Part model, mm, in its own coordinate system. Coordinates: 2 decimals unless noted, no trailing zeros. Order: outer loops, then holes, each group sorted by start corner. A loop starts at its lowest first (then second) coordinate and runs counter-clockwise, first axis right, second up. Notation, with made-up numbers: (-4, 64) - (51, 64) arc R15 cw to (51, 69) - close; hole circle Ø5 at (3.25, 24). An arc over 180 degrees is marked (long way). Use a Markdown table: item, result. Add a question column.
1) Saw through at D-D on y = 2.55. Count the separate pieces of the cut face and the enclosed holes in it, then the cut area to 3 significant figures.
2) Saw through at C-C on x = -42. List the corners of the cut face in (y, z).
3) Saw through at B-B on z = 20. List the corners of the cut face in (x, y), then the cut area to 3 significant figures.
4) Wall check: L1, parallel to Z at x = 22, y = 0.15; L2, parallel to X at y = 0.8, z = 25.5; L3, parallel to X at y = 2.4, z = -24. Give the ranges that are in metal, low to high. Write a range as [from, to].
5) Saw through at A-A on x = 22. List the corners of the cut face in (y, z).
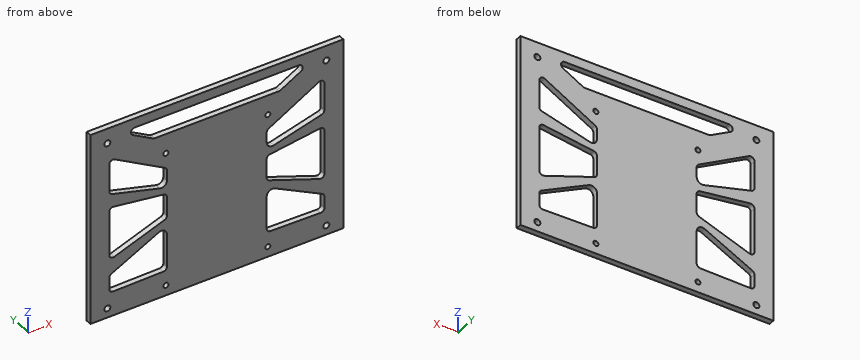
```python
from build123d import *

# Parameters (mm, degrees)
SKETCH_1_W          = 134
SKETCH_1_H          = 103
EXTRUDE_1_DEPTH     = 3
SKETCH_5_R          = 1.35
CUT_EXTRUDE_3_DEPTH = 85.559150895
SKETCH_6_R          = 1.6
CUT_EXTRUDE_4_DEPTH = 85.559150895
CUT_EXTRUDE_5_DEPTH = 85.559150895
FILLET_1_R          = 3
CUT_EXTRUDE_6_DEPTH = 85.559150895
FILLET_2_R          = 2


with BuildPart() as part:
    # 草图1 → 凸台-拉伸1 (new body)
    with BuildSketch(Plane(origin=(0, 0, 0), x_dir=(1, 0, 0), z_dir=(0, 1, 0))):
        Rectangle(SKETCH_1_W, SKETCH_1_H)
    extrude(amount=EXTRUDE_1_DEPTH)

    # 草图5 → 切除-拉伸3 (cut, through all)
    with BuildSketch(Plane(origin=(0, 3, 0), x_dir=(1, 0, 0), z_dir=(0, 1, 0))):
        with Locations(Location((27, -26, 0), (0, 0, 270))):
            Circle(SKETCH_5_R)
        with Locations(Location((-27, -26, 0), (0, 0, 270))):
            Circle(SKETCH_5_R)
        with Locations(Location((27, 46, 0), (0, 0, 270))):
            Circle(SKETCH_5_R)
        with Locations(Location((-27, 46, 0), (0, 0, 270))):
            Circle(SKETCH_5_R)
    extrude(amount=-CUT_EXTRUDE_3_DEPTH, mode=Mode.SUBTRACT)

    # 草图6 → 切除-拉伸4 (cut, through all)
    with BuildSketch(Plane(origin=(0, 3, 0), x_dir=(1, 0, 0), z_dir=(0, 1, 0))):
        with Locations(Location((58, 46.5, 0), (0, 0, 270))):
            Circle(SKETCH_6_R)
        with Locations(Location((58, -43.5, 0), (0, 0, 270))):
            Circle(SKETCH_6_R)
        with Locations(Location((-58, 46.5, 0), (0, 0, 90))):
            Circle(SKETCH_6_R)
        with Locations(Location((-58, -43.5, 0), (0, 0, 90))):
            Circle(SKETCH_6_R)
    extrude(amount=-CUT_EXTRUDE_4_DEPTH, mode=Mode.SUBTRACT)

    # 草图7 → 切除-拉伸5 (cut, through all)
    with BuildSketch(Plane.XZ):
        Polygon((-26.4206829, 17.634605341), (-57, 34.897123059), (-57, 15.273103969), (-26.4206829, 7.079400646), align=None)
        Polygon((-26.4206829, 3.713184828), (-57, 8.010827578), (-57, -20.746303353), (-26.4206829, -9.616342144), align=None)
        Polygon((-26.4206829, -37.989615661), (-26.4206829, -13.46201033), (-57, -29.042950621), (-57, -38.482830453), align=None)
        Polygon((57, -29.042950621), (26.4206829, -13.46201033), (26.4206829, -37.989615661), (57, -38.482830453), align=None)
        Polygon((26.4206829, 3.713184828), (26.4206829, -9.616342144), (57, -20.746303353), (57, 8.010827578), align=None)
        Polygon((26.4206829, 17.634605341), (26.4206829, 7.079400646), (57, 15.273103969), (57, 34.897123059), align=None)
    extrude(amount=-CUT_EXTRUDE_5_DEPTH, mode=Mode.SUBTRACT)

    # 圆角1
    fillet_1_edges = [part.edges().sort_by_distance(p)[0] for p in [
        (-26.4206829, 1.5, 7.079400646),
        (-26.4206829, 1.5, -13.46201033),
        (26.4206829, 1.5, -13.46201033),
        (26.4206829, 1.5, 7.079400646),
    ]]
    fillet(fillet_1_edges, radius=FILLET_1_R)

    # 草图9 → 切除-拉伸6 (cut, through all)
    with BuildSketch(Plane.XZ):
        Polygon((51.109101135, 46.5), (33.394815421, 36.5), (-33.394815421, 36.5), (-51.109101135, 46.5), align=None)
    extrude(amount=-CUT_EXTRUDE_6_DEPTH, mode=Mode.SUBTRACT)

    # 圆角2
    fillet_2_edges = [part.edges().sort_by_distance(p)[0] for p in [
        (-57, 1.5, 15.273103969),
        (-57, 1.5, 34.897123059),
        (-26.4206829, 1.5, 17.634605341),
        (-51.109101135, 1.5, 46.5),
        (51.109101135, 1.5, 46.5),
        (33.394815421, 1.5, 36.5),
        (-33.394815421, 1.5, 36.5),
        (-26.4206829, 1.5, -37.989615661),
        (-57, 1.5, -38.482830453),
        (-57, 1.5, -29.042950621),
        (-26.4206829, 1.5, -9.616342144),
        (-57, 1.5, -20.746303353),
        (-57, 1.5, 8.010827578),
        (-26.4206829, 1.5, 3.713184828),
        (26.4206829, 1.5, 3.713184828),
        (57, 1.5, 8.010827578),
        (57, 1.5, -20.746303353),
        (26.4206829, 1.5, -9.616342144),
        (57, 1.5, -29.042950621),
        (57, 1.5, -38.482830453),
        (26.4206829, 1.5, -37.989615661),
        (26.4206829, 1.5, 17.634605341),
        (57, 1.5, 34.897123059),
        (57, 1.5, 15.273103969),
    ]]
    fillet(fillet_2_edges, radius=FILLET_2_R)


solid = part.part
```
Results are:
| question | item | result |
|---|---|---|
| 1 | separate pieces | 1 |
| 1 | enclosed holes | 15 |
| 1 | area | 9,710 mm2 |
| 2 | outline | (0, -51.5) - (3, -51.5) - (3, -38.24) - (0, -38.24) - close; (0, -21.4) - (3, -21.4) - (3, -15.29) - (0, -15.29) - close; (0, 5.9) - (3, 5.9) - (3, 11.25) - (0, 11.25) - close; (0, 26.43) - (3, 26.43) - (3, 41.36) - (0, 41.36) - close; (0, 46.5) - (3, 46.5) - (3, 51.5) - (0, 51.5) - close |
| 3 | outline | (-67, 0) - (-57, 0) - (-57, 3) - (-67, 3) - close; (-30.61, 0) - (30.61, 0) - (30.61, 3) - (-30.61, 3) - close; (57, 0) - (67, 0) - (67, 3) - (57, 3) - close |
| 3 | area | 244 mm2 |
| 4 | L1 | [-51.5, 36.5], [46.5, 51.5] |
| 4 | L2 | [-67, -57], [-40.35, -28.25], [-25.75, 25.75], [28.25, 40.35], [57, 67] |
| 4 | L3 | [-67, -47.1], [-26.42, 26.42], [47.1, 67] |
| 5 | outline | (0, -51.5) - (3, -51.5) - (3, 36.5) - (0, 36.5) - close; (0, 46.5) - (3, 46.5) - (3, 51.5) - (0, 51.5) - close |
